Design review of the part built by this model. Coordinates are the model's own, in mm. Round coordinates to 2 decimals unless told otherwise and drop trailing zeros. Loops run counter-clockwise (first coordinate to the right, second up) from the corner with the lowest first, then second, coordinate; pieces in that order, holes last. Notation, with made-up numbers: (27.25, 49.5) -> (84.25, 49.5) arc R24 ccw to (84.25, 59.5) -> close; hole circle Ø5 at (78, 50). An arc over 180 degrees is marked (long way). Answer as CSV lines item,"result". Start each with the question number.
```python
from build123d import *

# Parameters (mm, degrees)
SKETCH1_R           = 1.25
BOSS_EXTRUDE1_DEPTH = 2
SKETCH2_R           = 2.45
SKETCH2_R_2         = 1.25
BOSS_EXTRUDE2_DEPTH = 1.34
FILLET1_R           = 0.6
CHAMFER1_SIZE       = 0.3


with BuildPart() as part:
    # Sketch1 → Boss-Extrude1 (new body)
    with BuildSketch(Plane.XY):
        Polygon((-1.41450816, 2.45), (1.41450816, 2.45), (2.829016319, 0), (1.41450816, -2.45), (-1.41450816, -2.45), (-2.829016319, 0), align=None)
        Circle(SKETCH1_R, mode=Mode.SUBTRACT)
    extrude(amount=BOSS_EXTRUDE1_DEPTH)

    # Sketch2 → Boss-Extrude2 (add)
    with BuildSketch(Plane.XY.offset(2)):
        Circle(SKETCH2_R)
        Circle(SKETCH2_R_2, mode=Mode.SUBTRACT)
    extrude(amount=BOSS_EXTRUDE2_DEPTH)

    # Fillet1
    fillet1_edges = [part.edges().sort_by_distance(p)[0] for p in [
        (-2.45, 0, 3.34),
    ]]
    fillet(fillet1_edges, radius=FILLET1_R)

    # Sketch3 → Cut-Revolve1 (revolve, cut)
    with BuildSketch(Plane(origin=(0, 0, 0), x_dir=(0, 0, -1), z_dir=(1, 0, 0))):
        Polygon((-2, 2.45), (-1.750031536, 2.95), (-0.249968464, 2.95), (0, 2.45), (0, 3.373191212), (-2, 3.373191212), align=None)
    revolve(axis=Axis((0, 0, 0), (0, 0, -1)), mode=Mode.SUBTRACT)

    # Chamfer1
    chamfer1_edges = [part.edges().sort_by_distance(p)[0] for p in [
        (-1.25, 0, 0),
    ]]
    chamfer(chamfer1_edges, length=CHAMFER1_SIZE)


solid = part.part
```
Q1. Mouldability with a two-part tool opening along X and no side actions: class faces 1 (the conical face through (-1.31, 2.26, 0.08)), 2 (the conical face through (1.287, 2.241, 1.933)), 3 (the cylindrical face through (-0.27, -1.22, 1.8)) as pulls with the +X half, pulls with the -X half, needs draft (parallel to the pull), parting line crosses it, or undercut.
Q2. Add section A-A, the plane z = 1.45. Give the boundary of the cut face in (x, y), and give its area (3 significant figures).
Q3. Add section B-B, the plane z = 3.1. Give the boundary of the cut face in (x, y).
Q4. For pin 1 Ø2 at (x, y) = (0, 0) entering from +Z; pin 2 Ø1.5 at (y, z) = (-1.5, 2) entering from -X, all flat-tipped, find the tip position at first contact; note any pin that passes through.
Q5. Add section C-C, the plane z = 2.65. Give the boundary of the cut face in (x, y), and give its area (3 significant figures).
Q6. To check wall thickness, follow probe 1 along Y at (x, z) = (0, 2.3); probe 2 along X at (y, z) = (-0.8, 2.1); probe 3 along Y at (x, z) = (0.5, 2.5). State the ranges of each line that lie inside material, in increasing order. Write a range as from..to.
Worked answers:
1,face 1,"pulls with the -X half"
1,face 2,"pulls with the +X half"
1,face 3,"undercut"
2,outline,"(-2.83, 0) -> (-1.41, -2.45) -> (1.41, -2.45) -> (2.83, 0) -> (1.41, 2.45) -> (-1.41, 2.45) -> close; hole circle Ø2.5 at (0, 0)"
2,area,"15.9 mm^2"
3,outline,"circle Ø4.66 at (0, 0); hole circle Ø2.5 at (0, 0)"
4,pin 1,"passes through"
4,pin 2,"stops at x = -2.4"
5,outline,"circle Ø4.9 at (0, 0); hole circle Ø2.5 at (0, 0)"
5,area,"13.9 mm^2"
6,probe 1,"y = -2.45..-1.25, 1.25..2.45"
6,probe 2,"x = -2.32..-0.96, 0.96..2.32"
6,probe 3,"y = -2.4..-1.15, 1.15..2.4"
